Could you check a few things on this model? Use its own coordinates, in mm. A direction names the side the tool comes from. Round coordinates to 2 decimals unless told otherwise and drop trailing zeros. Loops run counter-clockwise (first coordinate to the right, second up) from the corner with the lowest first, then second, coordinate; pieces in that order, holes last. Notation, with made-up numbers: (8, -9.75) -> (44, -9.75) arc R22 cw to (44, 23.25) -> close; hole circle Ø5 at (10.25, 44.25). An arc over 180 degrees is marked (long way). Put each result on its own line as item: value. Start each with the question number.
1. Which directions (+Z, -Z, +X, -X, +Y, -Y) give clear straight access to the entire face, cutting with the end or side of a thin tool? Please do faces 1 (the cylindrical face through (10.355, 0.986, -1.183)), 2 (the flat face through (2, 5, -3)), 3 (the cylindrical face through (-15, 7.5, 3.2)), 4 (the flat face through (2, 3.5, 0)).
2. Imagine slicing it at A-A, the plane y = 7.5. Please give me the cut outline in (x, z), and give its area (3 significant figures).
3. I'm going to push flat-ended pins straight in: P1, Ø4.5, axis at x = -20.5, y = 8.5, coming from the -Z side; P2, Ø2, axis at x = 4, z = 0.5, coming from the +Y side; P3, Ø5, axis at y = 9, z = -5.5, coming from the -X side. Where does each tip first touch, or does it pass through?
4. Imagine slicing it at D-D, the plane z = -0.75. Please give me the cut outline in (x, y).
5. Imagine slicing it at B-B, the plane z = 4.5. Please give me the cut outline in (x, y).
6. I need wall thicknesses on line 1 (X direction, y = 0.6, z = 0); line 2 (X direction, y = 4.2, z = 0); line 3 (Z direction, x = 8.5, y = 4.1). Which ranges of each line are inside material? Lowest first, please. Write a range as [from, to].
7. If we mould it in two halves opening along X, with no side actions, what happens to faces 5 (the flat face through (-25, 4, 2.5)), 6 (the flat face through (-9, 10, 0)), 7 (the flat face through (-25, 8, 4))? For each: pulls with the +X half, pulls with the -X half, needs draft (parallel to the pull), parting line crosses it, or undercut.
8. Imagine slicing it at C-C, the plane x = -31.5. Please give me the cut outline in (y, z), and give its area (3 significant figures).
```python
from build123d import *

# Parameters (mm, degrees)
SKETCH_1_W                   = 28
SKETCH_1_H                   = 15
EXTRUDE_1_DEPTH              = 5
SKETCH_2_W                   = 5
SKETCH_2_H                   = 15
EXTRUDE_2_DEPTH              = 10
SKETCH_3_W                   = 5
SKETCH_3_H                   = 15
EXTRUDE_3_DEPTH              = 23
CUT_EXTRUDE_1_DEPTH          = 1.5
HOLE_WIZARD_M2_1_D           = 2.4
HOLE_WIZARD_M2_1_CBORE_D     = 4.4
HOLE_WIZARD_M2_1_CBORE_DEPTH = 2
CUT_EXTRUDE_2_DEPTH          = 1.5


with BuildPart() as part:
    # 草图1 → 凸台-拉伸1 (new body)
    with BuildSketch(Plane(origin=(0, 0, 0), x_dir=(1, 0, 0), z_dir=(0, 1, 0))):
        Rectangle(SKETCH_1_W, SKETCH_1_H)
    extrude(amount=EXTRUDE_1_DEPTH)

    # 草图2 → 凸台-拉伸2 (add)
    with BuildSketch(Plane(origin=(0, 5, 0), x_dir=(1, 0, 0), z_dir=(0, 1, 0))):
        with Locations((-11.5, 0)):
            Rectangle(SKETCH_2_W, SKETCH_2_H)
    extrude(amount=EXTRUDE_2_DEPTH)

    # 草图3 → 凸台-拉伸3 (add)
    with BuildSketch(Plane.ZY.offset(14)):
        with Locations((5, 7.5)):
            Rectangle(SKETCH_3_W, SKETCH_3_H)
    extrude(amount=EXTRUDE_3_DEPTH)

    # 草图4 → 切除-拉伸1 (cut)
    with BuildSketch(Plane(origin=(0, 5, 0), x_dir=(1, 0, 0), z_dir=(0, 1, 0))):
        with BuildLine():
            Line((-6, 2), (6.697224362, 3))
            ThreePointArc((6.697224362, 3), (12, 0), (6.697224362, -3))
            Line((6.697224362, -3), (-6, -2))
            ThreePointArc((-6, -2), (-8, 0), (-6, 2))
        make_face()
    extrude(amount=-CUT_EXTRUDE_1_DEPTH, mode=Mode.SUBTRACT)

    # M2 凹头盖螺钉的柱形沉头孔1 (through all)
    with Locations(Plane(origin=(8.5, 0, 0), x_dir=(0, 0, -1), z_dir=(0, -1, 0))):
        with Locations((0, 0)):
            CounterBoreHole(HOLE_WIZARD_M2_1_D / 2, HOLE_WIZARD_M2_1_CBORE_D / 2, HOLE_WIZARD_M2_1_CBORE_DEPTH)

    # 草图7 → 切除-拉伸2 (cut)
    with BuildSketch(Plane(origin=(0, 0, 2.5), x_dir=(-1, 0, 0), z_dir=(0, 0, -1))):
        with BuildLine():
            Line((17, 9.5), (29.697224362, 10.5))
            ThreePointArc((29.697224362, 10.5), (35, 7.5), (29.697224362, 4.5))
            Line((29.697224362, 4.5), (17, 5.5))
            ThreePointArc((17, 5.5), (15, 7.5), (17, 9.5))
        make_face()
    extrude(amount=-CUT_EXTRUDE_2_DEPTH, mode=Mode.SUBTRACT)


solid = part.part
```
Entries:
1. face 1: -Y
1. face 2: +Z, -Z, +X, +Y
1. face 3: -Z
1. face 4: +Y
2. outline: (-37, 2.5) -> (-35, 2.5) -> (-35, 4) -> (-15, 4) -> (-15, 2.5) -> (-14, 2.5) -> (-14, -7.5) -> (-9, -7.5) -> (-9, 7.5) -> (-37, 7.5) -> close
2. area: 160 mm^2
3. P1: z = 2.5
3. P2: y = 3.5
3. P3: x = -14
4. outline: (-14, 0) -> (6.43, 0) -> (6.43, 2) -> (7.56, 2) -> (7.56, 3.5) -> (-7.85, 3.5) -> (-7.85, 5) -> (-9, 5) -> (-9, 15) -> (-14, 15) -> close; (9.44, 2) -> (10.57, 2) -> (10.57, 0) -> (14, 0) -> (14, 5) -> (11.92, 5) -> (11.92, 3.5) -> (9.44, 3.5) -> close
5. outline: (-37, 0) -> (14, 0) -> (14, 5) -> (-9, 5) -> (-9, 15) -> (-37, 15) -> close
6. line 1: [-14, 6.3], [10.7, 14]
6. line 2: [-14, -8], [12, 14]
6. line 3: [-7.5, -3.5], [3.5, 7.5]
7. face 5: needs draft
7. face 6: pulls with the +X half
7. face 7: undercut
8. outline: (0, 2.5) -> (4, 2.5) -> (4, 4) -> (11, 4) -> (11, 2.5) -> (15, 2.5) -> (15, 7.5) -> (0, 7.5) -> close
8. area: 64.5 mm^2
